```python
from build123d import *

# Parameters (mm, degrees)
SKETCH1_W               = 25
SKETCH1_H               = 63
BOSS_EXTRUDE1_DEPTH     = 4
SKETCH3_W               = 63
SKETCH3_H               = 4
BOSS_EXTRUDE2_DEPTH     = 2
SKETCH4_W               = 2
SKETCH4_H               = 63
BOSS_EXTRUDE3_DEPTH     = 61
SKETCH6_W               = 10
SKETCH6_H               = 2.5
CUT_EXTRUDE1_DEPTH      = 94.909530933
SKETCH6_3_W             = 10
SKETCH6_3_H             = 2.5
CUT_EXTRUDE2_DEPTH      = 80
SKETCH8_W               = 15
SKETCH8_H               = 2
CUT_EXTRUDE3_DEPTH      = 2.5
CUT_EXTRUDE5_DEPTH      = 15
SKETCH11_W              = 15
SKETCH11_H              = 2
CUT_EXTRUDE6_DEPTH      = 3
CUT_EXTRUDE7_DEPTH      = 15
FILLET6_R               = 2
FILLET7_R               = 2
BOSS_EXTRUDE4_DEPTH     = 53
FILLET8_R               = 0.4
FILLET9_R               = 2
CUT_EXTRUDE8_DEPTH      = 94.909530933
CUT_EXTRUDE8_DEPTH_BACK = 2
SKETCH15_W              = 11
SKETCH15_H              = 8


# Some blends are built 0.0001 mm under size
with BuildPart() as part:
    # Sketch1 → Boss-Extrude1 (new body)
    with BuildSketch(Plane(origin=(0, 0, 0), x_dir=(1, 0, 0), z_dir=(0, 1, 0))):
        with Locations((-12.5, -31.5)):
            Rectangle(SKETCH1_W, SKETCH1_H)
    extrude(amount=BOSS_EXTRUDE1_DEPTH)

    # Sketch3 → Boss-Extrude2 (add)
    with BuildSketch(Plane(origin=(0, 0, 0), x_dir=(0, 0, -1), z_dir=(1, 0, 0))):
        with Locations((-31.5, 2)):
            Rectangle(SKETCH3_W, SKETCH3_H)
    extrude(amount=BOSS_EXTRUDE2_DEPTH)

    # Sketch4 → Boss-Extrude3 (add)
    with BuildSketch(Plane(origin=(0, 4, 0), x_dir=(1, 0, 0), z_dir=(0, 1, 0))):
        with Locations((1, -31.5)):
            Rectangle(SKETCH4_W, SKETCH4_H)
    extrude(amount=BOSS_EXTRUDE3_DEPTH)

    # Sketch6 → Cut-Extrude1 (cut, through all)
    with BuildSketch(Plane.XZ):
        with Locations((-12, 1.25)):
            Rectangle(SKETCH6_W, SKETCH6_H)
    extrude(amount=-CUT_EXTRUDE1_DEPTH, mode=Mode.SUBTRACT)

    # Sketch6<3> → Cut-Extrude2 (cut)
    with BuildSketch(Plane.XZ):
        with Locations((-12, 61.75)):
            Rectangle(SKETCH6_3_W, SKETCH6_3_H)
    extrude(amount=-CUT_EXTRUDE2_DEPTH, mode=Mode.SUBTRACT)

    # Sketch8 → Cut-Extrude3 (cut)
    with BuildSketch(Plane.XY.offset(63)):
        with Locations((-12, 1)):
            Rectangle(SKETCH8_W, SKETCH8_H)
    extrude(amount=-CUT_EXTRUDE3_DEPTH, mode=Mode.SUBTRACT)

    # Sketch9 → Cut-Extrude5 (cut)
    with BuildSketch(Plane.ZY.offset(4.5)):
        with BuildLine():
            ThreePointArc((61.5, 2.5), (61, 2.366025404), (60.633974596, 2))
            Line((60.633974596, 2), (63, 2))
            Line((63, 2), (61.5, 2.5))
        make_face()
    extrude(amount=CUT_EXTRUDE5_DEPTH, mode=Mode.SUBTRACT)

    # Sketch11 → Cut-Extrude6 (cut)
    with BuildSketch(Plane(origin=(0, 0, 0), x_dir=(-1, 0, 0), z_dir=(0, 0, -1))):
        with Locations((12, 1)):
            Rectangle(SKETCH11_W, SKETCH11_H)
    extrude(amount=-CUT_EXTRUDE6_DEPTH, mode=Mode.SUBTRACT)

    # Sketch12 → Cut-Extrude7 (cut)
    with BuildSketch(Plane.ZY.offset(4.5)):
        with BuildLine():
            ThreePointArc((2.766025404, 2), (2.4, 2.366025404), (1.9, 2.5))
            Line((1.9, 2.5), (0, 2))
            Line((0, 2), (2.766025404, 2))
        make_face()
    extrude(amount=CUT_EXTRUDE7_DEPTH, mode=Mode.SUBTRACT)

    # Fillet6
    fillet6_edges = [part.edges().sort_by_distance(p)[0] for p in [
        (-19.5, 0, 1.5),
        (-22.25, 0, 0),
        (-25, 0, 31.5),
        (-22.25, 0, 63),
        (-19.5, 0, 61.75),
        (-12, 0, 60.5),
        (-4.5, 0, 61.75),
        (-1.25, 0, 63),
        (2, 0, 31.5),
        (-1.25, 0, 0),
        (-4.5, 0, 1.5),
        (-12, 0, 3),
    ]]
    fillet(fillet6_edges, radius=FILLET6_R - 0.0001)  # a hair under: the kernel refuses the full size

    # Fillet7
    # the kernel refuses this fillet: 2 mm, written as the material it takes off along each edge
    with BuildSketch(Plane(origin=(-23, 0, 61), x_dir=(0, 0, 1), z_dir=(1, 0, 0))) as fillet7_piece_1:
        with BuildLine():
            CenterArc((0.0001, -1.9999), 1.9999, 0, 90)
            Line((2, -1.9999), (2, 0))
            Line((2, 0), (0.0001, 0))
        make_face()
    revolve(axis=Axis((-23, 0, 61), (0, -1, 0)), revolution_arc=90, mode=Mode.SUBTRACT)
    with BuildSketch(Plane(origin=(-23, 0, 2), x_dir=(-1, 0, 0), z_dir=(0, 0, 1))) as fillet7_piece_2:
        with BuildLine():
            CenterArc((0.0001, -1.9999), 1.9999, 0, 90)
            Line((2, -1.9999), (2, 0))
            Line((2, 0), (0.0001, 0))
        make_face()
    revolve(axis=Axis((-23, 0, 2), (0, -1, 0)), revolution_arc=90, mode=Mode.SUBTRACT)
    with BuildSketch(Plane(origin=(-25, 0, 63), x_dir=(0, 0, -1), z_dir=(0, 1, 0)), Plane(origin=(-25, 0, 0), x_dir=(1, 0, 0), z_dir=(0, 1, 0))) as fillet7_piece_3:
        with BuildLine():
            CenterArc((FILLET7_R, -FILLET7_R), FILLET7_R, 90, 90)
            Line((0, -FILLET7_R), (0, 0))
            Line((0, 0), (FILLET7_R, 0))
        make_face()
    extrude(amount=9, mode=Mode.SUBTRACT)

    # Sketch13 → Boss-Extrude4 (add)
    with BuildSketch(Plane(origin=(0, 4, 0), x_dir=(1, 0, 0), z_dir=(0, 1, 0))):
        Polygon((0, -4.25), (-1.5, -4.25), (-1.5, -2.6), (-2.7, -2.6), (-2.7, -5.6), (0, -5.6), align=None)
        Polygon((-1.5, -60.4), (-2.7, -60.4), (-2.7, -57.4), (0, -57.4), (0, -58.75), (-1.5, -58.75), align=None)
    extrude(amount=BOSS_EXTRUDE4_DEPTH)

    # Fillet8
    fillet8_edges = [part.edges().sort_by_distance(p)[0] for p in [
        (0, 30.5, 5.6),
        (-1.5, 4, 3.425),
        (-2.1, 4, 2.6),
        (-1.5, 30.5, 2.6),
        (-2.7, 4, 4.1),
        (-2.7, 30.5, 2.6),
        (-1.35, 4, 5.6),
        (-2.7, 30.5, 5.6),
        (0, 57, 4.925),
        (-2.1, 57, 2.6),
        (-2.7, 57, 4.1),
        (-1.35, 57, 5.6),
        (-1.5, 4, 59.575),
        (-1.5, 30.5, 60.4),
        (-1.35, 4, 57.4),
        (0, 30.5, 57.4),
        (-2.7, 4, 58.9),
        (-2.7, 30.5, 57.4),
        (-2.1, 4, 60.4),
        (-2.7, 30.5, 60.4),
        (0, 57, 58.075),
        (-1.35, 57, 57.4),
        (-2.7, 57, 58.9),
        (-2.1, 57, 60.4),
    ]]
    fillet(fillet8_edges, radius=FILLET8_R)

    # Fillet9
    # the kernel refuses this fillet: 2 mm, written as the material it takes off along each edge
    with BuildSketch(Plane(origin=(0, 0, 61), x_dir=(1, 0, 0), z_dir=(0, 0, -1))) as fillet9_piece_1:
        with BuildLine():
            CenterArc((0.0001, -1.9999), 1.9999, 0, 90)
            Line((2, -1.9999), (2, 0))
            Line((2, 0), (0.0001, 0))
        make_face()
    revolve(axis=Axis((0, 0, 61), (0, -1, 0)), revolution_arc=90, mode=Mode.SUBTRACT)
    with BuildSketch(Plane(origin=(0, 0, 2), x_dir=(0, 0, -1), z_dir=(-1, 0, 0))) as fillet9_piece_2:
        with BuildLine():
            CenterArc((0.0001, -1.9999), 1.9999, 0, 90)
            Line((2, -1.9999), (2, 0))
            Line((2, 0), (0.0001, 0))
        make_face()
    revolve(axis=Axis((0, 0, 2), (0, -1, 0)), revolution_arc=90, mode=Mode.SUBTRACT)
    with BuildSketch(Plane(origin=(0, 63, 61), x_dir=(0, 0, 1), z_dir=(1, 0, 0))) as fillet9_piece_3_section:
        Polygon((0, 0), (FILLET9_R, 0), (FILLET9_R, -FILLET9_R), (0, -FILLET9_R), align=None)
    fillet9_piece_3 = extrude(amount=FILLET9_R, mode=Mode.PRIVATE)
    fillet9_piece_3 = fillet9_piece_3 - Plane(origin=(0, 63, 61), x_dir=(0, -0.7071067811865475, -0.7071067811865475), z_dir=(1, 0, 0)) * Sphere(FILLET9_R, mode=Mode.PRIVATE)
    add(fillet9_piece_3, mode=Mode.SUBTRACT)
    with BuildSketch(Plane(origin=(0, 63, 2), x_dir=(0, 0, -1), z_dir=(0, 1, 0))) as fillet9_piece_4_section:
        Polygon((0, 0), (FILLET9_R, 0), (FILLET9_R, -FILLET9_R), (0, -FILLET9_R), align=None)
    fillet9_piece_4 = extrude(amount=FILLET9_R, mode=Mode.PRIVATE)
    fillet9_piece_4 = fillet9_piece_4 - Plane(origin=(0, 63, 2), x_dir=(-0.7071067811865474, 0, 0.7071067811865476), z_dir=(0, 1, 0)) * Sphere(FILLET9_R, mode=Mode.PRIVATE)
    add(fillet9_piece_4, mode=Mode.SUBTRACT)
    with BuildSketch(Plane(origin=(2, 63, 63), x_dir=(-1, 0, 0), z_dir=(0, -1, 0)), Plane(origin=(2, 63, 0), x_dir=(0, 0, 1), z_dir=(0, -1, 0))) as fillet9_piece_5:
        with BuildLine():
            CenterArc((FILLET9_R, FILLET9_R), FILLET9_R, 180, 90)
            Line((0, FILLET9_R), (0, 0))
            Line((0, 0), (FILLET9_R, 0))
        make_face()
    extrude(amount=63, mode=Mode.SUBTRACT)
    with BuildSketch(Plane(origin=(2, 65, 2), x_dir=(-1, 0, 0), z_dir=(0, 0, 1))) as fillet9_piece_6:
        with BuildLine():
            CenterArc((FILLET9_R, FILLET9_R), FILLET9_R, 180, 90)
            Line((0, FILLET9_R), (0, 0))
            Line((0, 0), (FILLET9_R, 0))
        make_face()
    extrude(amount=59, mode=Mode.SUBTRACT)
    with BuildSketch(Plane(origin=(-5, 65, 0), x_dir=(0, 0, 1), z_dir=(1, 0, 0))) as fillet9_piece_7:
        with BuildLine():
            CenterArc((FILLET9_R, FILLET9_R), FILLET9_R, 180, 90)
            Line((0, FILLET9_R), (0, 0))
            Line((0, 0), (FILLET9_R, 0))
        make_face()
    extrude(amount=5, mode=Mode.SUBTRACT)
    with BuildSketch(Plane(origin=(0, 65, 63), x_dir=(0, -1, 0), z_dir=(-1, 0, 0))) as fillet9_piece_8:
        with BuildLine():
            CenterArc((FILLET9_R, -FILLET9_R), FILLET9_R, 90, 90)
            Line((0, -FILLET9_R), (0, 0))
            Line((0, 0), (FILLET9_R, 0))
        make_face()
    extrude(amount=5, mode=Mode.SUBTRACT)

    # Sketch15 → Cut-Extrude8 (cut, two sides: drawn at the far end of the back side and taken through both)
    with BuildSketch(Plane(origin=(0, 0, 0), x_dir=(-1, 0, 0), z_dir=(0, -1, 0)).offset(-CUT_EXTRUDE8_DEPTH_BACK)):
        with Locations((11.5, -42.5)):
            Rectangle(SKETCH15_W, SKETCH15_H)
        Polygon((22, -31.625), (17, -38.5), (6, -38.5), (1, -31.625), align=None)
        with BuildLine():
            ThreePointArc((15.742640687, -27.382359313), (11.5, -25.625), (7.257359313, -27.382359313))
            ThreePointArc((7.257359313, -27.382359313), (7.257359313, -28.796572875), (8.671572875, -28.796572875))
            ThreePointArc((8.671572875, -28.796572875), (11.5, -27.625), (14.328427125, -28.796572875))
            ThreePointArc((14.328427125, -28.796572875), (15.742640687, -28.796572875), (15.742640687, -27.382359313))
        make_face()
        with BuildLine():
            ThreePointArc((18.864708263, -24.14094547), (11.415609445, -21.125339137), (4.01594547, -24.260291737))
            ThreePointArc((4.01594547, -24.260291737), (4.027311781, -25.674459622), (5.441479666, -25.663093311))
            ThreePointArc((5.441479666, -25.663093311), (11.431683837, -23.12527454), (17.461906689, -25.566479666))
            ThreePointArc((17.461906689, -25.566479666), (18.876074574, -25.555113355), (18.864708263, -24.14094547))
        make_face()
        with BuildLine():
            ThreePointArc((22.106601718, -21.018398282), (11.5, -16.625), (0.893398282, -21.018398282))
            ThreePointArc((0.893398282, -21.018398282), (0.893398282, -22.432611845), (2.307611845, -22.432611845))
            ThreePointArc((2.307611845, -22.432611845), (11.5, -18.625), (20.692388155, -22.432611845))
            ThreePointArc((20.692388155, -22.432611845), (22.106601718, -22.432611845), (22.106601718, -21.018398282))
        make_face()
    extrude(amount=CUT_EXTRUDE8_DEPTH + CUT_EXTRUDE8_DEPTH_BACK, mode=Mode.SUBTRACT)


solid = part.part
```
CAD build for the part. Positions are in the model's coordinates, mm. A direction names the side the tool comes from. Round coordinates to 2 decimals unless told otherwise and drop trailing zeros. Order: outer loops, then holes, each group sorted by start corner. A loop starts at its lowest first (then second) coordinate and runs counter-clockwise, first axis right, second up. Notation, with made-up numbers: (-14, -32.5) - (-2, -32.5) arc R37 ccw to (-2, 4.5) - close; hole circle Ø9 at (-28, -22.5). An arc over 180 degrees is marked (long way). Answer in a Markdown table with one row per item. Add a question column.
(1) Band-saw the part on B-B on y = 33.5. List the corners of the cut face in (x, z).
(2) Band-saw the part on A-A on z = 7. List the corners of the cut face in (x, y), and give its area (3 significant figures).
(3) Mould opens along X. For faces 4 (the face through (2, 32, 32)), 5 (the face through (-3.535, 1.014, 35.111)), 6 (the face through (-4.012, 1.014, 25.659)), 7 (the face through (-20, 3, 63)) say: +X half, -X half, draft (parallel to the pull), parting line (faces both ways), or undercut.
(4) Band-saw the part on D-D on z = 41. List the corners of the cut face in (x, y), and give its area (3 significant figures).
(5) 3-axis set-ups, long thin cutter, end or side, ignore diameter. For faces 1 (the face through (-17, 3, 1)), 2 (the face through (-3.93, 0.6, 61.22)), 3 (the face through (-11.357, 1.014, 18.626)): which of +Z, -Z, +X, -X, +Y, -Y reach the whole face in a straight line?
(6) Drop flat-ended pins along their axis: pin 1 Ø0.6 at (y, z) = (3.5, 61.5) entering from -X; pin 2 Ø1 at (x, z) = (-1.5, 3.5) entering from +Y; pin 3 Ø4 at (x, z) = (-10.5, 44) entering from +Y. Give the stop position or say it passes through.
(7) Probe L1, parallel to Z at x = -0.75, y = 22; L2, parallel to Y at x = -15.5, z = 19.5; L3, parallel to X at y = 19.5, z = 60. List the from-to ranges inside material, lowest first. Write a range as [from, to].
Data:
| question | item | result |
|---|---|---|
| 1 | outline | (-2.7, 3) arc R0.4 ccw to (-2.3, 2.6) - (-1.9, 2.6) arc R0.4 ccw to (-1.5, 3) - (-1.5, 4.25) - (0, 4.25) - (0, 0) arc R2 ccw to (2, 2) - (2, 61) arc R2 ccw to (0, 63) - (0, 58.75) - (-1.5, 58.75) - (-1.5, 60) arc R0.4 ccw to (-1.9, 60.4) - (-2.3, 60.4) arc R0.4 ccw to (-2.7, 60) - (-2.7, 57.8) arc R0.4 ccw to (-2.3, 57.4) - (-0.4, 57.4) arc R0.4 cw to (0, 57) - (0, 6) arc R0.4 cw to (-0.4, 5.6) - (-2.3, 5.6) arc R0.4 ccw to (-2.7, 5.2) - close |
| 2 | outline | (-25, 2) arc R2 ccw to (-23, 0) - (0, 0) arc R2 ccw to (2, 2) - (2, 63) arc R2 ccw to (0, 65) - (0, 4) - (-25, 4) - close |
| 2 | area | 227 mm^2 |
| 3 | face 4 | +X half |
| 3 | face 5 | undercut |
| 3 | face 6 | undercut |
| 3 | face 7 | draft |
| 4 | outline | (-25, 2) arc R2 ccw to (-23, 0) - (-17, 0) - (-17, 2) - (-6, 2) - (-6, 0) - (0, 0) arc R2 ccw to (2, 2) - (2, 63) arc R2 ccw to (0, 65) - (0, 4) - (-25, 4) - close |
| 4 | area | 205 mm^2 |
| 5 | face 1 | -Z, +Y, -Y |
| 5 | face 2 | +Z, -Y |
| 5 | face 3 | -Y |
| 6 | pin 1 | stops at x = -24.99 |
| 6 | pin 2 | stops at y = 57 |
| 6 | pin 3 | stops at y = 4 |
| 7 | L1 | z = [4.25, 5.6], [57.4, 58.75] |
| 7 | L2 | y = [0, 4] |
| 7 | L3 | x = [-2.7, -1.5], [0, 2] |
